Read the model definition and answer for the solid it produces. Units are mm, in the model's axes. A direction names the side the tool comes from. Give positions to 0.01 mm unless a question says otherwise; leave off trailing zeros. Write each loop counter-clockwise with the first axis right and the second up, starting at its lowest first coordinate (ties: lowest second). Pieces come first, ordered by that corner, then holes. Notation, with made-up numbers: (43.25, 25.25) -> (67.25, 25.25) arc R23 ccw to (67.25, 57.25) -> close; hole circle Ø5 at (-36, 17.25). An arc over 180 degrees is marked (long way). Put each result on its own line as item: value. Start each with the question number.
Autodesk Fusion 360 part; units mm, degrees
sketch "スケッチ1" plane through (0, 0, 0) normal (0, 1, 0) x (1, 0, 0)
  circle A0 centre (0, 0) radius 3.5
  circle A1 centre (0, 0) radius 8
  dimension "d1" = 7
  dimension "d14" = 16
extrude "押し出し1" add sketch "スケッチ1" along normal blind 15 contours A0 makes body 1
extrude "押し出し2" add sketch "スケッチ1" against normal blind 2 contours A0 | A1 bodies 1
sphere "球プリミティブ1" add diameter 34 placed x (1, 0, 0) y (0, 0, -1) z (0, 1, 0) at (0, 0, 0) separate body makes body 2
move_body "移動1" bodies 2 to x (1, 0, 0) y (0, 1, 0) z (0, 0, 1) at (0, 38.5, 0)
fillet "フィレット4" radius 1 1 edges at (-3.2631, 0, 1.2657) on bodies 1
fillet "フィレット5" radius 1 1 edges at (-3.2631, 15, 1.2657) on bodies 1
fillet "フィレット6" radius 1 2 edges at (-7.4586, 0, 2.8929) (-7.4586, -2, -2.8929) on bodies 1
delete_body "RemoveBody1" bodies 2
1) A cutting plane is placed at C-C on y = 10.5. Give the vertices of the cut face in (x, z), and give its area (3 significant figures).
2) Each of these flat-tipped pins is pushed along its axis until it touches: pin 1 Ø1 at (y, z) = (11.5, 0.5) entering from +X; pin 2 Ø1 at (x, y) = (4.5, 9) entering from -Z; pin 3 Ø3 at (x, z) = (0.5, 6) entering from +Y; pin 4 Ø8 at (y, z) = (10.5, 4) entering from -X. Where does it stop, or does it pass through?
3) Straight lines are drawn through the part: line 1 (Y direction, x = 3, z = 5.25); line 2 (X direction, y = 0.5, z = -1); line 3 (X direction, y = 6, z = 1). For each, find the intervals that lie inside material, in ascending order. Write a range as [from, to].
4) For faces 1 (the face through (3.233, 7.409, -1.341)), 2 (the face through (0, 15, 0)), determine the directions among +Z, -Z, +X, -X, +Y, -Y from which every point of the face is accessible in a straight line to the end or side of a thin tool.
Results found:
1. outline: circle Ø7 at (0, 0)
1. area: 38.5 mm²
2. pin 1: stops at x = 3.5
2. pin 2: passes through
2. pin 3: stops at y = 0
2. pin 4: stops at x = -3.5
3. line 1: y = [-2, 0]
3. line 2: x = [-3.49, 3.49]
3. line 3: x = [-3.35, 3.35]
4. face 1: +Y
4. face 2: +Z, -Z, +X, -X, +Y
